from build123d import *

# Parameters (mm, degrees)
F1_DEPTH = 26.8
F3_DEPTH = 51.5
F4_W     = 13
F4_H     = 3
F5_DEPTH = 5
F6_W     = 1.5
F6_H     = 13
F7_DEPTH = 22.75
F8_W     = 10
F8_H     = 8.7
F9_DEPTH = 38.5


with BuildPart() as f1:
    # F0 (on Top) → F1 (new body)
    with BuildSketch(Plane.XY):
        Polygon((29.5, 51.5), (-29.5, 51.5), (-29.5, 0), (-5, 0), (-5, 13), (5, 13), (5, 0), (29.5, 0), align=None)
    extrude(amount=F1_DEPTH)

    # F2 (on face) → F3 (cut, through all)
    with BuildSketch(Plane.XZ):
        Polygon((10.242246, 26.8), (29.5, 0), (29.5, 26.8), align=None)
        Polygon((-29.5, 26.8), (-29.5, 0), (-10.242246, 26.8), align=None)
    extrude(amount=-F3_DEPTH, mode=Mode.SUBTRACT)

    # F4 (on face) → F5 (cut)
    with BuildSketch(Plane.XZ.offset(-13)):
        with Locations((0, 23.3)):
            Rectangle(F4_W, F4_H)
    extrude(amount=-F5_DEPTH, mode=Mode.SUBTRACT)

    # F6 (on face) → F7 (cut)
    with BuildSketch(Plane.XY.offset(26.8)):
        with Locations((-5.75, 6.5)):
            Rectangle(F6_W, F6_H)
        with Locations((5.75, 6.5)):
            Rectangle(F6_W, F6_H)
    extrude(amount=-F7_DEPTH, mode=Mode.SUBTRACT)

    # F8 (on face) → F9 (cut, through all)
    with BuildSketch(Plane.XZ.offset(-13)):
        with Locations((0, 4.35)):
            Rectangle(F8_W, F8_H)
    extrude(amount=-F9_DEPTH, mode=Mode.SUBTRACT)


solid = f1.part
Check sheet for the modelled part. Datum: model origin and axes. Units: mm. A direction names the side the tool comes from. Round coordinates to 2 decimals unless told otherwise and drop trailing zeros. Order: outer loops, then holes, each group sorted by start corner. A loop starts at its lowest first (then second) coordinate and runs counter-clockwise, first axis right, second up.
(1) Cross-section at D-D, the plane z = 19. Enter the section's corners in (x, y).
(2) Go/stop test with flat-tipped pins: P1, Ø2, axis at y = 15.5, z = 14.5, coming from the +X side; P2, Ø2.5, axis at x = 1, y = 15, coming from the -Z side; P3, Ø5, axis at x = 9, z = 4.5, coming from the -Y side; P4, Ø4.5, axis at y = 35, z = 3.5, coming from the -X side. Record where each tip stops, or that it passes through.
(3) Draft check along Z on faces 6 (the flat face through (0, 26, 26.8)), 7 (the flat face through (0, 32, 8.7)), 8 (the flat face through (0, 18, 23)). Enter one of: pulls with the +Z half, pulls with the -Z half, needs draft (parallel to the pull), parting line crosses it, or undercut.
(4) Access from +Z, -Z, +X, -X, +Y, -Y to the whole of each face (thin tool, end or side, straight path). Record for faces 1 (the flat face through (19.736, 25.39, 13.588)), 2 (the flat face through (0, 13, 26)), 3 (the flat face through (-5, 25, 4)), 4 (the flat face through (17, 26, 0)), 5 (the flat face through (0, 15, 21.8)).
(5) Cross-section at A-A, the plane y = 11. Enter the section's corners in (x, z), and give its area (3 significant figures).
(6) Scan lines: probe 1 along Z at (x, y) = (-2, 16.5); probe 2 along Y at (x, z) = (-2, 20.5); probe 3 along X at (y, z) = (29, 3.5) (3 decimals). Record each from-to range of solid material in increasing order.
(7) Cross-section at B-B, the plane y = 40.5. Enter the section's corners in (x, z).
(8) Cross-section at C-C, the plane z = 2. Enter the section's corners in (x, y), and give its area (3 significant figures).
Check sheet entries:
1. outline: (-15.85, 0) - (-6.5, 0) - (-6.5, 13) - (6.5, 13) - (6.5, 0) - (15.85, 0) - (15.85, 51.5) - (-15.85, 51.5) - close
2. P1: stops at x = 19.8
2. P2: stops at z = 8.7
2. P3: stops at y = 0
2. P4: stops at x = -28.6
3. face 6: pulls with the +Z half
3. face 7: pulls with the -Z half
3. face 8: undercut
4. face 1: +Z, +X, +Y, -Y
4. face 2: +Z, -Y
4. face 3: -Z, +Y, -Y
4. face 4: -Z, +X, -X, +Y, -Y
4. face 5: -Y
5. outline: (-29.5, 0) - (-5, 0) - (-5, 4.05) - (-6.5, 4.05) - (-6.5, 26.8) - (-10.24, 26.8) - close; (5, 0) - (29.5, 0) - (10.24, 26.8) - (6.5, 26.8) - (6.5, 4.05) - (5, 4.05) - close
5. area: 729 mm2
6. probe 1: z = 8.7 to 21.8, 24.8 to 26.8
6. probe 2: y = 13 to 51.5
6. probe 3: x = -26.985 to -5, 5 to 26.985
7. outline: (-29.5, 0) - (-5, 0) - (-5, 8.7) - (5, 8.7) - (5, 0) - (29.5, 0) - (10.24, 26.8) - (-10.24, 26.8) - close
8. outline: (-28.06, 0) - (-5, 0) - (-5, 51.5) - (-28.06, 51.5) - close; (5, 0) - (28.06, 0) - (28.06, 51.5) - (5, 51.5) - close
8. area: 2,380 mm2
